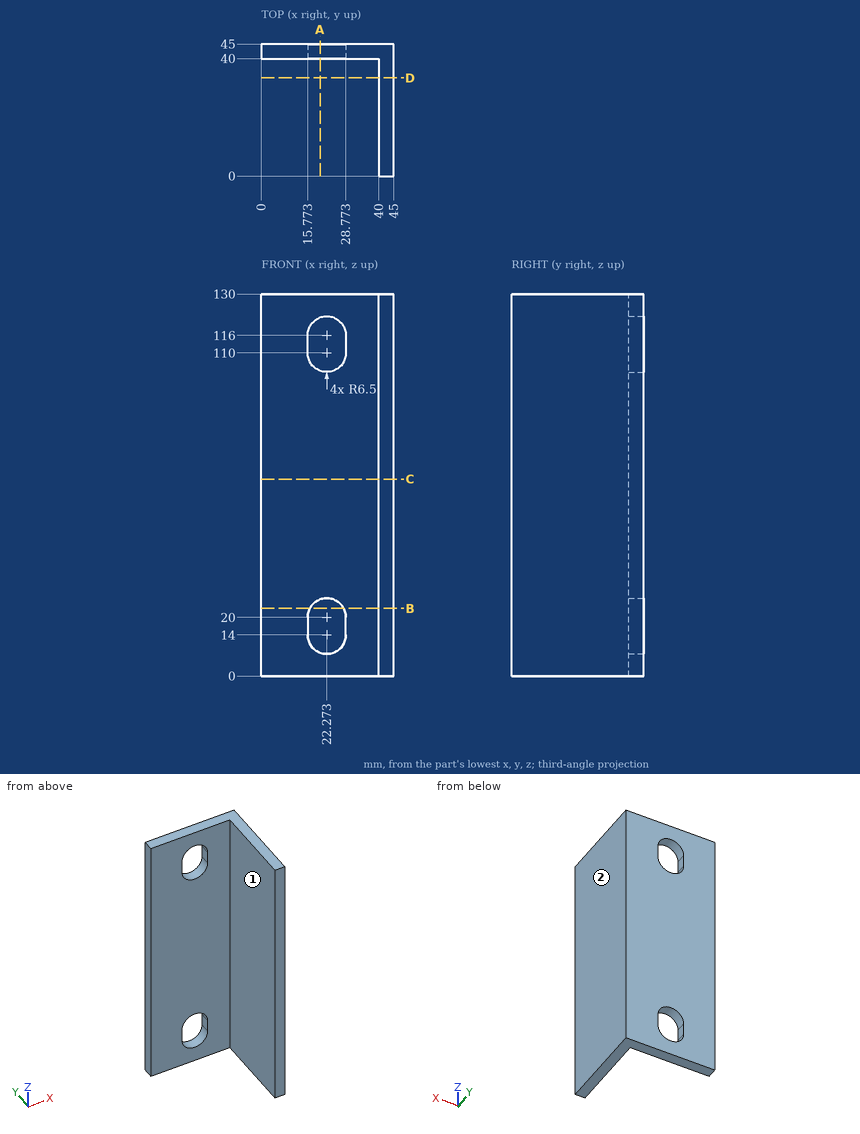
Geometry check sheet. Reference: drawing and pictorial views, mm from the part's lowest x, y, z. A direction names the side the tool comes from. Coordinates: 2 decimals unless noted, no trailing zeros. Loops run counter-clockwise (first coordinate to the right, second up) from the corner with the lowest first, then second, coordinate; pieces in that order, holes last. Notation, with made-up numbers: (8, 30) -> (50, 30) arc R35 cw to (50, 63) -> close; hole circle Ø2 at (53.5, 61). An arc over 180 degrees is marked (long way). Write item = value, one per line. Start each with the question number.
1. Tool access check on the marked faces 1 and 2. Record the directions out of +Z, -Z, +X, -X, +Y, -Y that give a thin tool (end or side, any length) a straight path to the whole face; none if there is none.
2. Section check C-C on z = 67. Record the cut outline in (x, y), then the cut area to 3 significant figures.
3. Material ranges on line 1 (Y direction, x = 2.5, z = 79), recorded low to high.
4. Section check B-B on z = 23. Record the cut outline in (x, y).
5. Section check D-D on y = 33.5. Record the cut outline in (x, z), then the cut area to 3 significant figures.
6. Depth check by flat-ended pin: P1, Ø10, axis at y = 27.5, z = 34.5, coming from the -X side; P2, Ø5, axis at x = 37, z = 101, coming from the -Y side. Enter the tip coordinate at first touch or a pass-through.
7. Section check A-A on x = 20. Record the cut outline in (y, z).
Responses:
q1.face_1 = +Z, -Z, -X, -Y
q1.face_2 = +Z, -Z, +X, +Y, -Y
q2.outline = (0, 40) -> (40, 40) -> (40, 0) -> (45, 0) -> (45, 45) -> (0, 45) -> close
q2.area = 425 mm2
q3.line_1 = 40 to 45
q4.outline = (0, 40) -> (16.51, 40) -> (16.51, 45) -> (0, 45) -> close; (28.04, 40) -> (40, 40) -> (40, 0) -> (45, 0) -> (45, 45) -> (28.04, 45) -> close
q5.outline = (40, 0) -> (45, 0) -> (45, 130) -> (40, 130) -> close
q5.area = 650 mm2
q6.P1 = 40
q6.P2 = 40
q7.outline = (40, 0) -> (45, 0) -> (45, 7.91) -> (40, 7.91) -> close; (40, 26.09) -> (45, 26.09) -> (45, 103.91) -> (40, 103.91) -> close; (40, 122.09) -> (45, 122.09) -> (45, 130) -> (40, 130) -> close
